Check sheet for the modelled part. Datum: model origin and axes. Units: mm. A direction names the side the tool comes from. Coordinates: 2 decimals unless noted, no trailing zeros. Write each loop counter-clockwise with the first axis right and the second up, starting at its lowest first coordinate (ties: lowest second). Pieces come first, ordered by that corner, then holes. Notation, with made-up numbers: (-26, -8.5) -> (19, -8.5) arc R12 ccw to (19, 0.5) -> close; hole circle Ø2 at (-19, 80). An arc over 180 degrees is marked (long way). Put each result on its own line as item: value.
```python
from build123d import *

# Parameters (mm, degrees)
F0_R     = 4.5
F0_R_2   = 2
F2_DEPTH = 3
F1_R     = 1.185
F3_DEPTH = 25
F4_DEPTH = 4.5


with BuildPart() as f2:
    # F0 (on Top) → F2 (new body)
    with BuildSketch(Plane.XY):
        with BuildLine():
            Line((-1.5, 12.409674), (-9, -8.674676))
            ThreePointArc((-9, -8.674676), (0, -12.5), (9, -8.674676))
            Line((9, -8.674676), (1.5, 12.409674))
            ThreePointArc((1.5, 12.409674), (0, 12.5), (-1.5, 12.409674))
        make_face()
        Circle(F0_R, mode=Mode.SUBTRACT)
        Circle(F0_R)
        Circle(F0_R_2, mode=Mode.SUBTRACT)
    extrude(amount=F2_DEPTH)

    # F1 (on Top) → F3 (cut)
    with BuildSketch(Plane.XY):
        with Locations((0, 9)):
            Circle(F1_R)
    extrude(amount=F3_DEPTH, mode=Mode.SUBTRACT)

    # F0 (on Top) → F4 (join)
    with BuildSketch(Plane.XY):
        Circle(F0_R)
        Circle(F0_R_2, mode=Mode.SUBTRACT)
    extrude(amount=F4_DEPTH)


solid = f2.part
```
Q1. Cross-section at B-B (y = 0). Record the cut outline in (x, z).
Recorded:
outline: (-5.91, 0) -> (-2, 0) -> (-2, 4.5) -> (-4.5, 4.5) -> (-4.5, 3) -> (-5.91, 3) -> close; (2, 0) -> (5.91, 0) -> (5.91, 3) -> (4.5, 3) -> (4.5, 4.5) -> (2, 4.5) -> close
Q2. Mould release check, pull along Y, two halves, no side actions. Record for faces 1 (the cylindrical face through (0, -2, 2)), 2 (the flat face through (2, -1, 4.5)), 3 (the cylindrical face through (-0.1, -12.5, 1.5)): released by +Y, released by -Y, zero draft, split by the parting line, or undercut.
Recorded:
face 1: undercut
face 2: zero draft
face 3: released by -Y
Q3. Cross-section at C-C (z = 1.35). Record the cut outline in (x, y) (3 decimals).
Recorded:
outline: (-9, -8.675) arc R12.5 ccw to (9, -8.675) -> (1.5, 12.41) arc R12.5 ccw to (-1.5, 12.41) -> close; hole circle Ø4 at (0, 0); hole circle Ø2.37 at (0, 9)
Q4. Material ranges on line 1 along Y through (x, z) = (0, 2.1) (3 decimals); line 2 along X through (y, z) = (10, 0.3); line 3 along Z through (x, y) = (5, -10), recorded low to high.
Recorded:
line 1: y = -12.5 to -2, 2 to 7.815, 10.185 to 12.5
line 2: x = -2.36 to -0.64, 0.64 to 2.36
line 3: z = 0 to 3
Q5. Cross-section at A-A (x = 0). Record the cut outline in (y, z) (3 decimals).
Recorded:
outline: (-12.5, 0) -> (-2, 0) -> (-2, 4.5) -> (-4.5, 4.5) -> (-4.5, 3) -> (-12.5, 3) -> close; (2, 0) -> (7.815, 0) -> (7.815, 3) -> (4.5, 3) -> (4.5, 4.5) -> (2, 4.5) -> close; (10.185, 0) -> (12.5, 0) -> (12.5, 3) -> (10.185, 3) -> close
Q6. Tool access check on faces 4 (the cylindrical face through (-0.59, 4.46, 3.74)), 5 (the cylindrical face through (-0.154, 10.175, 1.479)). Record the directions out of +Z, -Z, +X, -X, +Y, -Y that give a thin tool (end or side, any length) a straight path to the whole face; none if there is none.
Recorded:
face 4: +Z
face 5: +Z, -Z
Q7. Cross-section at D-D (z = 4.15). Record the cut outline in (x, y), plus the area to 3 significant figures.
Recorded:
outline: circle Ø9 at (0, 0); hole circle Ø4 at (0, 0)
area: 51.1 mm2
Q8. Depth check by flat-ended pin: P1, Ø1.5, axis at x = 4, y = -7, coming from the +Z side; P2, Ø5, axis at x = 0, y = 0, coming from the +Z side. Enter the tip coordinate at first touch or a pass-through.
Recorded:
P1: stops at z = 3
P2: stops at z = 4.5
